The figure shows three views and two pictorial views of one solid part (mm, origin at its lowest corner). Answer the questions. Give positions to 0.01 mm unless a question says otherwise; leave off trailing zeros. Loops run counter-clockwise (first coordinate to the right, second up) from the corner with the lowest first, then second, coordinate; pieces in that order, holes last. Notation, with made-up numbers: (74, 63.5) - (108, 63.5) arc R24 cw to (108, 88.5) - close; hole circle Ø10 at (54, -32). An arc over 180 degrees is marked (long way). Use a Markdown table: item, result. Add a question column.
Item 1: For a pull along Y with two mould halves and no side action, classify the marked faces 1 and 2 as +Y half, -Y half, draft (parallel to the pull), parting line (faces both ways), or undercut.
Item 2: Each of these flat-tipped pins is pushed along its axis until it touches: P1, Ø1, axis at y = 2.5, z = 28, coming from the +X side; P2, Ø6, axis at x = 13, z = 14.5, coming from the +Y side; P3, Ø3, axis at x = 5, z = 14, coming from the +Y side. Where does it stop, or does it pass through?
Item 3: A cutting plane is placed at C-C (z = 21). Determine the outline of the cut face in (x, y), plus the area to 3 significant figures.
Item 4: A cutting plane is placed at D-D (x = 24.5). Determine the outline of the cut face in (y, z).
Item 5: A cutting plane is placed at B-B (z = 16.75). Determine the outline of the cut face in (x, y).
Item 6: A cutting plane is placed at A-A (x = 16.75). Determine the outline of the cut face in (y, z), plus the area to 3 significant figures.
Item 7: Consider probe 1 along X at (y, z) = (1.15, 16.75); probe 2 along X at (y, z) = (0.8, 16.75); probe 3 along Z at (x, y) = (16.75, 1.15). Determine where each line is inside the solid, lowest interval first. Write a range as [from, to].
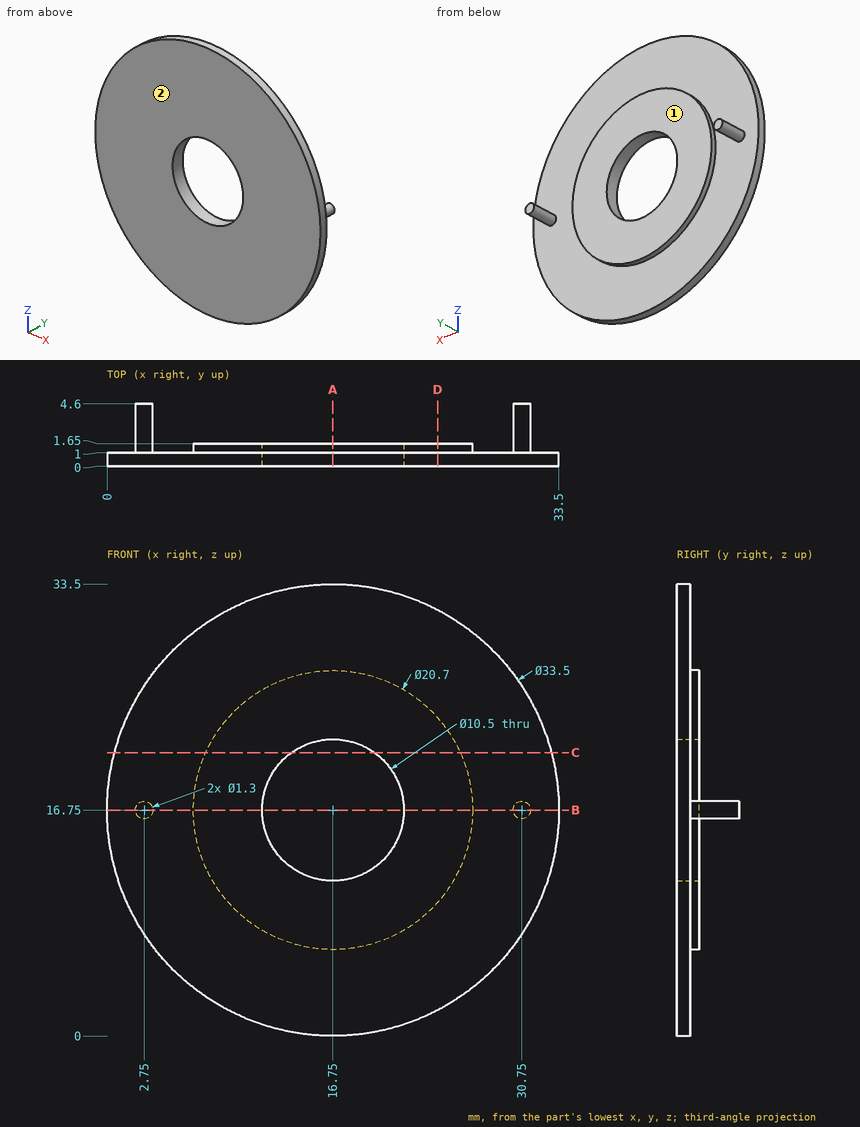
Geometry says:
| question | item | result |
|---|---|---|
| 1 | face 1 | +Y half |
| 1 | face 2 | -Y half |
| 2 | P1 | through |
| 2 | P2 | y = 1.65 |
| 2 | P3 | y = 1 |
| 3 | outline | (0.55, 0) - (13.67, 0) - (13.67, 1.65) - (7.31, 1.65) - (7.31, 1) - (0.55, 1) - close; (19.83, 0) - (32.95, 0) - (32.95, 1) - (26.19, 1) - (26.19, 1.65) - (19.83, 1.65) - close |
| 3 | area | 34.5 mm² |
| 4 | outline | (0, 1.9) - (1, 1.9) - (1, 9.89) - (1.65, 9.89) - (1.65, 23.61) - (1, 23.61) - (1, 31.6) - (0, 31.6) - close |
| 5 | outline | (0, 0) - (11.5, 0) - (11.5, 1.65) - (6.4, 1.65) - (6.4, 1) - (3.4, 1) - (3.4, 4.6) - (2.1, 4.6) - (2.1, 1) - (0, 1) - close; (22, 0) - (33.5, 0) - (33.5, 1) - (31.4, 1) - (31.4, 4.6) - (30.1, 4.6) - (30.1, 1) - (27.1, 1) - (27.1, 1.65) - (22, 1.65) - close |
| 6 | outline | (0, 0) - (1, 0) - (1, 6.4) - (1.65, 6.4) - (1.65, 11.5) - (0, 11.5) - close; (0, 22) - (1.65, 22) - (1.65, 27.1) - (1, 27.1) - (1, 33.5) - (0, 33.5) - close |
| 6 | area | 29.6 mm² |
| 7 | probe 1 | [2.1, 3.4], [6.4, 11.5], [22, 27.1], [30.1, 31.4] |
| 7 | probe 2 | [0, 11.5], [22, 33.5] |
| 7 | probe 3 | [6.4, 11.5], [22, 27.1] |
